Part model, mm, in its own coordinate system. A direction names the side the tool comes from. Round coordinates to 2 decimals unless told otherwise and drop trailing zeros. Loops run counter-clockwise (first coordinate to the right, second up) from the corner with the lowest first, then second, coordinate; pieces in that order, holes last.
(1) Tool access for faces 4 (the face through (0, 1, -10.75)), 5 (the face through (0, 0, 0)), 6 (the face through (3.36, 0.29, -9.21)), 7 (the face through (3.36, 2.71, -9.21)): list every direction of +Z, -Z, +X, -X, +Y, -Y with a clear straight run to the whole face (end or side of a thin tool).
(2) Flat gauge pin, fed straight in: pin 1 (3 mm diameter, centred on x = -14.5, z = 0, fed in from -Y). Where does the tip first touch, or does it go through?
(3) Mould opens along Z. For faces 1 (the face through (9.139, 1.485, -14.334)), 2 (the face through (0, 3, 0)), 3 (the face through (-3.36, 0.29, -9.29)) say: +Z half, -Z half, draft (parallel to the pull), parting line (faces both ways), or undercut.
(4) Cut at B-B on y = 1.95. List the corners of the cut face in (x, z), then the cut area to 3 significant figures.
(5) Probe probe 1 along X at (y, z) = (1.15, 0); probe 2 along Z at (x, y) = (-0.5, 0.4); probe 3 along Z at (x, y) = (-15, 2.8). List the from-to ranges inside material, lowest first.
(6) Cut at A-A on x = 0. List the corners of the cut face in (y, z).
from build123d import *

# Parameters (mm, degrees)
SKETCH1_R           = 17
SKETCH1_R_2         = 1.65
BOSS_EXTRUDE1_DEPTH = 3
CHAMFER1_SIZE       = 0.4


with BuildPart() as part:
    # Sketch1 → Boss-Extrude1 (new body)
    with BuildSketch(Plane(origin=(0, 0, 0), x_dir=(1, 0, 0), z_dir=(0, 1, 0))):
        Circle(SKETCH1_R)
        with Locations((-14.5, 0)):
            Circle(SKETCH1_R_2, mode=Mode.SUBTRACT)
        with Locations((14.5, 0)):
            Circle(SKETCH1_R_2, mode=Mode.SUBTRACT)
        with BuildLine():
            Line((-1.75, 7.75), (1.75, 7.75))
            ThreePointArc((1.75, 7.75), (3.25, 9.25), (1.75, 10.75))
            Line((1.75, 10.75), (-1.75, 10.75))
            ThreePointArc((-1.75, 10.75), (-3.25, 9.25), (-1.75, 7.75))
        make_face(mode=Mode.SUBTRACT)
    extrude(amount=BOSS_EXTRUDE1_DEPTH)

    # Chamfer1
    chamfer1_edges = [part.edges().sort_by_distance(p)[0] for p in [
        (-3.25, 3, -9.25),
        (0, 3, -7.75),
        (-16.15, 0, 0),
        (-16.15, 3, 0),
        (-17, 0, 0),
        (12.85, 0, 0),
        (12.85, 3, 0),
        (-17, 3, 0),
        (3.25, 0, -9.25),
        (0, 0, -10.75),
        (-3.25, 0, -9.25),
        (0, 0, -7.75),
        (3.25, 3, -9.25),
        (0, 3, -10.75),
    ]]
    chamfer(chamfer1_edges, length=CHAMFER1_SIZE)


solid = part.part
Final values:
1. face 4: +Y, -Y
1. face 5: +Z, -Z, +X, -X, -Y
1. face 6: -Y
1. face 7: +Y
2. pin 1: passes through
3. face 1: parting line
3. face 2: draft
3. face 3: undercut
4. outline: circle Ø34 at (0, 0); hole circle Ø3.3 at (-14.5, 0); hole (-1.75, -10.75) - (1.75, -10.75) arc R1.5 ccw to (1.75, -7.75) - (-1.75, -7.75) arc R1.5 ccw to start; hole circle Ø3.3 at (14.5, 0)
4. area: 873 mm2
5. probe 1: x = -17 to -16.15, -12.85 to 12.85, 16.15 to 17
5. probe 2: z = -16.99 to -10.75, -7.75 to 16.99
5. probe 3: z = -7.57 to -1.78, 1.78 to 7.57
6. outline: (0, -16.6) - (0.4, -17) - (2.6, -17) - (3, -16.6) - (3, -11.15) - (2.6, -10.75) - (0.4, -10.75) - (0, -11.15) - close; (0, -7.35) - (0.4, -7.75) - (2.6, -7.75) - (3, -7.35) - (3, 16.6) - (2.6, 17) - (0.4, 17) - (0, 16.6) - close
